Build history of the part. All positions in model axes, mm. A direction names the side the tool comes from. Give positions to 0.01 mm unless a question says otherwise; leave off trailing zeros. Loops run counter-clockwise (first coordinate to the right, second up) from the corner with the lowest first, then second, coordinate; pieces in that order, holes last. Notation, with made-up numbers: (54.5, 76) -> (109.5, 76) arc R17 ccw to (109.5, 101) -> close; hole circle Ø7 at (71.25, -19.5). An arc over 180 degrees is marked (long way). Answer in a Markdown table with one row per item. Add a question column.
Solid Edge part; units mm, degrees
sketch "Sketch1" plane through (0, 0, 0) normal (0, -1, 0) x (1, 0, 0)
  line L0 (0, 0) -> (19.9, 0)
  line L1 (19.9, 0) -> (19.9, 7.8)
  line L2 (19.9, 7.8) -> (0, 7.8)
  line L3 (0, 7.8) -> (0, 0)
  dimension "D1" = 19.9
extrude "Protrusion1" add sketch "Sketch1" against normal blind 7.8
sketch "Sketch2" plane through (19.9, 3.95, 3.95) normal (1, 0, 0) x (0, 1, 0)
  line L0 (3.85, 3.85) -> (-3.95, 3.85)
  line L1 (-3.95, 3.85) -> (-3.95, -0.95)
  line L2 (-3.95, -0.95) -> (-0.95, -3.95)
  line L3 (-0.95, -3.95) -> (0.85, -3.95)
  line L4 (0.85, -3.95) -> (3.85, -0.95)
  line L5 (3.85, -0.95) -> (3.85, 3.85)
extrude "ExtrudedProtrusion_2" add sketch "Sketch2" along normal blind 60
fillet "Round_1" radius 15 1 edges at (79.9, 3.9, 0)
(1) Saw through at B-B, the plane z = 2.25. List the corners of the cut face in (x, y).
(2) 3-axis set-ups, long thin cutter, end or side, ignore diameter. For faces 1 (the flat face through (47.4, 6.3, 1.5)), 2 (the flat face through (47, 1, 2)), 3 (the flat face through (41, 7.8, 5)): which of +Z, -Z, +X, -X, +Y, -Y reach the whole face in a straight line?
(3) Flat gauge pins, fed straight in: pin 1 Ø2 at (x, z) = (21.5, 1) entering from -Y; pin 2 Ø1.5 at (y, z) = (1, 1.5) entering from +X; pin 3 Ø0.9 at (y, z) = (5.5, 1.5) entering from +X. Where does each tip first touch, or does it go through?
(4) Saw through at C-C, the plane y = 3.75. List the corners of the cut face in (x, z).
(5) Saw through at D-D, the plane y = 0.75. List the corners of the cut face in (x, z), then the cut area to 3 significant figures.
(6) Saw through at A-A, the plane x = 60.5. List the corners of the cut face in (y, z).
(7) Wall check: line 1 along X through (y, z) = (1.25, 3); line 2 along X through (y, z) = (7.25, 2); line 3 along Z through (x, y) = (68, 5). Give the ranges that are in metal, low to high. Write a range as from..to.
Worked answers:
| question | item | result |
|---|---|---|
| 1 | outline | (0, 0) -> (19.9, 0) -> (19.9, 0.75) -> (74.64, 0.75) -> (74.64, 7.05) -> (19.9, 7.05) -> (19.9, 7.8) -> (0, 7.8) -> close |
| 2 | face 1 | -Z, +X, +Y |
| 2 | face 2 | -Z, +X, -Y |
| 2 | face 3 | +Z, -Z, +X, -X, +Y |
| 3 | pin 1 | y = 1 |
| 3 | pin 2 | x = 74.64 |
| 3 | pin 3 | x = 74.14 |
| 4 | outline | (0, 0) -> (66.74, 0) arc R15 ccw to (79.9, 7.8) -> (0, 7.8) -> close |
| 5 | outline | (0, 0) -> (19.9, 0) -> (19.9, 2.25) -> (74.64, 2.25) arc R15 ccw to (79.9, 7.8) -> (0, 7.8) -> close |
| 5 | area | 476 mm^2 |
| 6 | outline | (0, 3) -> (3, 0) -> (4.8, 0) -> (7.8, 3) -> (7.8, 7.8) -> (0, 7.8) -> close |
| 7 | line 1 | 0..75.74 |
| 7 | line 2 | 0..19.9 |
| 7 | line 3 | 0.2..7.8 |
